Read the model definition and answer for the solid it produces. Units are mm, in the model's axes. Face numbers are marked on the shaded views. A direction names the side the tool comes from. Give positions to 0.01 mm unless a question says otherwise; leave off trailing zeros. Write each loop counter-clockwise with the first axis right and the second up, starting at its lowest first coordinate (ties: lowest second). Pieces come first, ordered by that corner, then holes. Notation, with made-up numbers: M 13,-5 L 18,-5 A20 ccw 18,8 Z; hole C 25,-23.75 d8. An arc over 180 degrees is marked long. Use a Markdown table: item, result. Add a question column.
Item 1: Consider probe 1 along Z at (x, y) = (-83, 0); probe 2 along Z at (x, y) = (-63, 0); probe 3 along X at (y, z) = (-2.25, -50.5). Determine where each line is inside the solid, lowest interval first. Write a range as [from, to].
Item 2: The mould has two halves that part along Z. Classify the marked faces 1, 2, 3 and 4: pulls with the +Z half, pulls with the -Z half, needs draft (parallel to the pull), parting line crosses it, or undercut.
Item 3: A cutting plane is placed at C-C on z = -34. Determine the outline of the cut face in (x, y), then the cut area to 3 significant figures.
Item 4: A cutting plane is placed at D-D on x = -92.5. Determine the outline of the cut face in (y, z), then the cut area to 3 significant figures.
Item 5: For the marked faces 5 and 6, determine the directions among +Z, -Z, +X, -X, +Y, -Y from which every point of the face is accessible in a straight line to the end or side of a thin tool.
Item 6: A cutting plane is placed at B-B on x = -81.5. Determine the outline of the cut face in (y, z), then the cut area to 3 significant figures.
Item 7: Given P1, Ø8, axis at x = -44.5, z = -29.5, coming from the +Y side; P2, Ø5, axis at y = 1.5, z = -56.5, coming from the -X side; P3, Ø4.5, axis at x = -82, y = 1.5, coming from the -Z side; P4, Ø4, axis at y = -3, z = -72, coming from the +X side, each flat-ended and moving along its own axis, determine where each tip first touches the part or whether it passes through.
Item 8: A cutting plane is placed at A-A on y = -1.5. Determine the outline of the cut face in (x, z).
from build123d import *

# Parameters (mm, degrees)
BOSS_EXTRUDE1_DEPTH = 4.5


with BuildPart() as part:
    # Sketch1 → Boss-Extrude1 (new, symmetric)
    with BuildSketch(Plane(origin=(0, 0, 0), x_dir=(1, 0, 0), z_dir=(0, 1, 0))):
        with BuildLine():
            Line((-101.508620324, 2), (-67.260686883, 2))
            ThreePointArc((-67.260686883, 2), (-62.036309634, 3.941462028), (-59.347664897, 8.823529412))
            ThreePointArc((-59.347664897, 8.823529412), (-51.737318493, 30.385027154), (-36.613340144, 47.533812423))
            ThreePointArc((-36.613340144, 47.533812423), (-33.647401917, 52.31816148), (-34.5669156, 57.87165408))
            Line((-34.5669156, 57.87165408), (-51.667108069, 87.490056256))
            ThreePointArc((-51.667108069, 87.490056256), (-56.868026794, 91.301361412), (-63.19102199, 90.038295963))
            ThreePointArc((-63.19102199, 90.038295963), (-94.99085495, 55.468346611), (-109.470080741, 10.784313725))
            ThreePointArc((-109.470080741, 10.784313725), (-107.436288913, 4.627594105), (-101.508620324, 2))
        make_face()
        with BuildLine():
            Line((-53.583601177, 60.80951969), (-55.668486055, 64.420646227))
            ThreePointArc((-55.668486055, 64.420646227), (-61.622662682, 68.361129347), (-68.352706691, 65.97656772))
            Line((-68.352706691, 65.97656772), (-90.993256658, 27.298850575))
            ThreePointArc((-90.993256658, 27.298850575), (-89.749031081, 20.224584028), (-83.330666624, 17))
            Line((-83.330666624, 17), (-79.14543575, 17))
            ThreePointArc((-79.14543575, 17), (-74.41664671, 18.547205705), (-71.516960015, 22.590361446))
            Line((-71.516960015, 22.590361446), (-54.679341331, 51.333903335))
            ThreePointArc((-54.679341331, 51.333903335), (-52.564762349, 55.890540621), (-53.583601177, 60.80951969))
        make_face(mode=Mode.SUBTRACT)
    extrude(amount=BOSS_EXTRUDE1_DEPTH, both=True)


solid = part.part
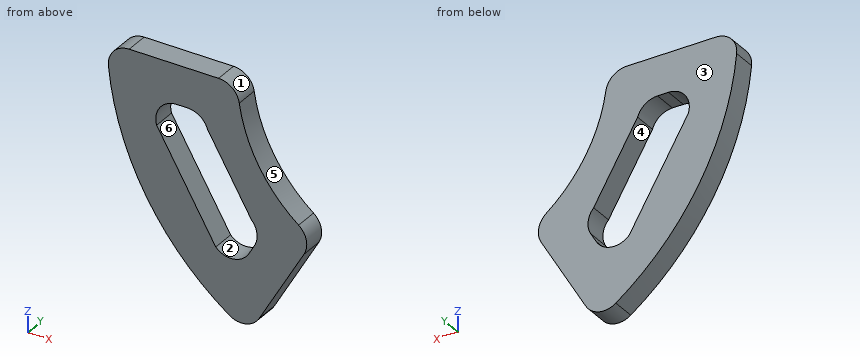
Filled in:
| question | item | result |
|---|---|---|
| 1 | probe 1 | [-72.19, -40.95], [-17, -2] |
| 1 | probe 2 | [-90.17, -68.41], [-37.13, -3.23] |
| 1 | probe 3 | [-97.72, -77.41], [-55.17, -34.24] |
| 2 | face 1 | pulls with the +Z half |
| 2 | face 2 | undercut |
| 2 | face 3 | needs draft |
| 2 | face 4 | undercut |
| 3 | outline | M -104.61,-4.5 L -87.07,-4.5 L -87.07,4.5 L -104.61,4.5 Z; M -64.83,-4.5 L -49.44,-4.5 L -49.44,4.5 L -64.83,4.5 Z |
| 3 | area | 296 mm² |
| 4 | outline | M -4.5,-59.53 L 4.5,-59.53 L 4.5,-2 L -4.5,-2 Z |
| 4 | area | 518 mm² |
| 5 | face 5 | +Z, +X, +Y, -Y |
| 5 | face 6 | +Y, -Y |
| 6 | outline | M -4.5,-73.88 L 4.5,-73.88 L 4.5,-43.52 L -4.5,-43.52 Z; M -4.5,-17 L 4.5,-17 L 4.5,-2 L -4.5,-2 Z |
| 6 | area | 408 mm² |
| 7 | P1 | through |
| 7 | P2 | x = -95.83 |
| 7 | P3 | z = -75.76 |
| 7 | P4 | x = -41.57 |
| 8 | outline | M -109.47,-10.78 A110 ccw -63.19,-90.04 A8 ccw -51.67,-87.49 L -34.57,-57.87 A8 ccw -36.61,-47.53 A60 cw -59.35,-8.82 A8 ccw -67.26,-2 L -101.51,-2 A8 ccw Z; hole M -90.99,-27.3 L -68.35,-65.98 A8 ccw -55.67,-64.42 L -53.58,-60.81 A8 ccw -54.68,-51.33 L -71.52,-22.59 A8 ccw -79.15,-17 L -83.33,-17 A8 ccw Z |
